For this review, use the dimensioned drawing (mm, ordinates from the lowest corner) and the shaded views. Give positions to 0.01 mm unless a question says otherwise; leave off trailing zeros. Loops run counter-clockwise (first coordinate to the right, second up) from the corner with the lowest first, then second, coordinate; pieces in that order, holes last. Notation, with made-up numbers: M 69,56 L 88,56 A11 ccw 88,66 Z; hole C 17,60.5 d11. An arc over 180 degrees is marked long. Use CSV: the item, a comma, the result in double quotes. Start each with the question number.
1. Take a section at D-D, the plane x = 8. Write out the cut boundary in (y, z).
2. To check wall thickness, follow line 1 (X direction, y = 3.25, z = 43); line 2 (Z direction, x = 40, y = 6.75); line 3 (Z direction, x = 53.5, y = 6). State the ranges of each line that lie inside material, in increasing order. Write a range as [from, to].
3. The part is to be moulded in two halves that separate along X. For the marked faces 1, 2, 3 and 4, say which applies: pulls with the +X half, pulls with the -X half, needs draft (parallel to the pull), parting line crosses it, or undercut.
4. Take a section at B-B, the plane y = 5.75. Write out the cut boundary in (x, z), and give its area (3 significant figures).
5. Take a section at C-C, the plane z = 62. Write out the cut boundary in (x, y).
6. Take a section at A-A, the plane z = 35. Write out the cut boundary in (x, y), and give its area (3 significant figures).
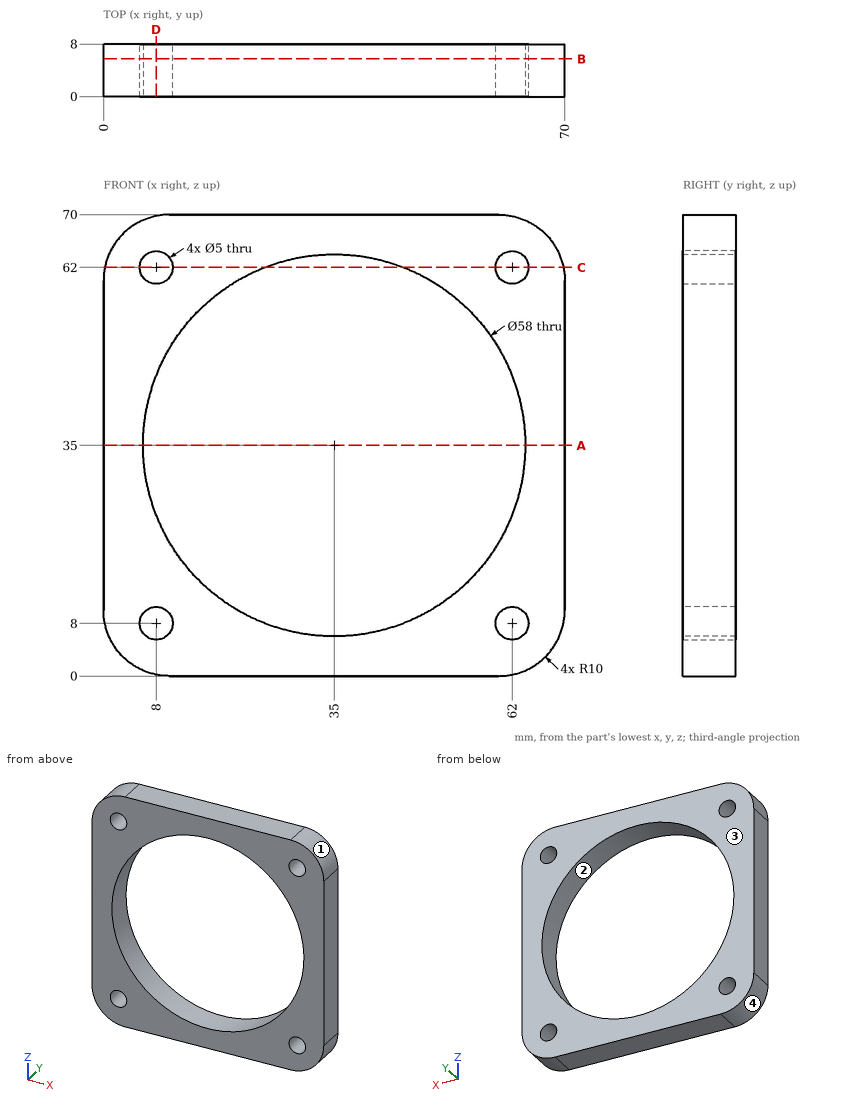
Result set:
1,outline,"M 0,0.2 L 8,0.2 L 8,5.5 L 0,5.5 Z; M 0,10.5 L 8,10.5 L 8,24.42 L 0,24.42 Z; M 0,45.58 L 8,45.58 L 8,59.5 L 0,59.5 Z; M 0,64.5 L 8,64.5 L 8,69.8 L 0,69.8 Z"
2,line 1,"[0, 7.13], [62.87, 70]"
2,line 2,"[0, 6.43], [63.57, 70]"
2,line 3,"[0, 12.67], [57.33, 70]"
3,face 1,"pulls with the +X half"
3,face 2,"undercut"
3,face 3,"needs draft"
3,face 4,"pulls with the -X half"
4,outline,"M 0,10 A10 ccw 10,0 L 60,0 A10 ccw 70,10 L 70,60 A10 ccw 60,70 L 10,70 A10 ccw 0,60 Z; hole C 8,8 d5; hole C 8,62 d5; hole C 35,35 d58; hole C 62,8 d5; hole C 62,62 d5"
4,area,"2,090 mm2"
5,outline,"M 0.2,0 L 5.5,0 L 5.5,8 L 0.2,8 Z; M 10.5,0 L 24.42,0 L 24.42,8 L 10.5,8 Z; M 45.58,0 L 59.5,0 L 59.5,8 L 45.58,8 Z; M 64.5,0 L 69.8,0 L 69.8,8 L 64.5,8 Z"
6,outline,"M 0,0 L 6,0 L 6,8 L 0,8 Z; M 64,0 L 70,0 L 70,8 L 64,8 Z"
6,area,"96.0 mm2"
